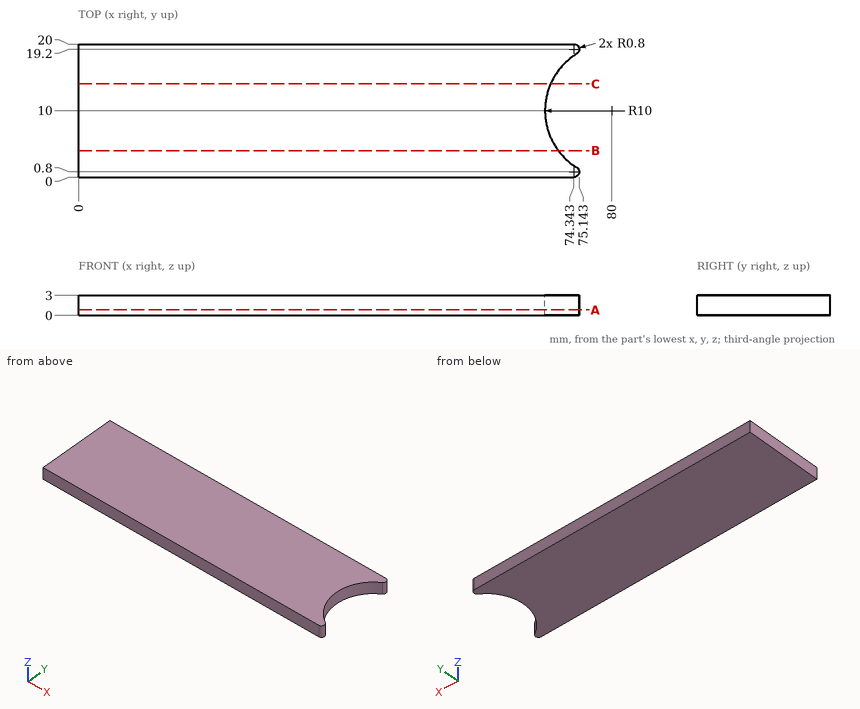
Can you work these out from the drawing? Everything is in mm from the part's minimum corner. Give positions to 0.01 mm unless a question says otherwise; leave off trailing zeros. Order: outer loops, then holes, each group sorted by start corner. A loop starts at its lowest first (then second) coordinate and runs counter-clockwise, first axis right, second up. Notation, with made-up numbers: M 48.5,-16.5 L 52.5,-16.5 A19 cw 52.5,17.5 Z; hole C 60,40 d8. An arc over 180 degrees is marked long. Use a Markdown table: item, result. Add a question column.
Item 1: If I drill on L1, parallel to X at y = 6, z = 0.2 (1 decimal); L2, parallel to X at y = 4, z = 0.25, over which ranges is the centre line in solid material (lowest first)? Write a range as [from, to].
Item 2: Suppose I cut it at C-C (y = 14). List the corners of the cut face in (x, z) for me (3 decimals), then the cut area to 4 significant figures.
Item 3: Suppose I cut it at A-A (z = 0.8). List the corners of the cut face in (x, y) for me, then the cut area to 3 significant figures.
Item 4: Suppose I cut it at B-B (y = 4). List the corners of the cut face in (x, z) for me.
Answer sheet:
| question | item | result |
|---|---|---|
| 1 | L1 | x = [0, 70.8] |
| 1 | L2 | x = [0, 72] |
| 2 | outline | M 0,0 L 70.835,0 L 70.835,3 L 0,3 Z |
| 2 | area | 212.5 mm² |
| 3 | outline | M 0,0 L 74.34,0 A0.8 ccw 74.76,1.48 A10 cw 74.76,18.52 A0.8 ccw 74.34,20 L 0,20 Z |
| 3 | area | 1,440 mm² |
| 4 | outline | M 0,0 L 72,0 L 72,3 L 0,3 Z |
